Input: dimensioned drawing with shaded views. Units: mm. Origin: part minimum x, y, z. Round coordinates to 2 decimals unless told otherwise and drop trailing zeros. Order: outer loops, then holes, each group sorted by start corner. A loop starts at its lowest first (then second) coordinate and runs counter-clockwise, first axis right, second up. Notation, with made-up numbers: M 25,88.25 L 82,88.25 A29 ccw 82,125.25 Z; hole C 57,33.25 d5. An arc over 180 degrees is marked long. Use one line per item in the form item = value. Start each with the question number.
Q1. Material intervals for probe 1 along Z at (x, y) = (123, 2.15); probe 2 along Z at (x, y) = (79, 1.2) (1 decimal); probe 3 along X at (y, z) = (2.5, 35.5) (1 decimal), sorted ascending.
Q2. Section A-A (z = 95.25). Give the number of separate pieces and of enclosed holes in the cut face, plus the area to 3 significant figures.
Q3. Contact query for flat-ended pins moving along their axis: pin 1 (1 mm diameter, centred on x = 131.5, y = 2, fed in from -Z); pin 2 (1.6 mm diameter, centred on y = 1.5, z = 70, fed in from -X) (3 decimals); pin 3 (1 mm diameter, centred on x = 2, y = 2, fed in from +Z). Output: stop coordinate, or through.
Q4. Section B-B (x = 59). Return the cut outline in (y, z) (1 decimal).
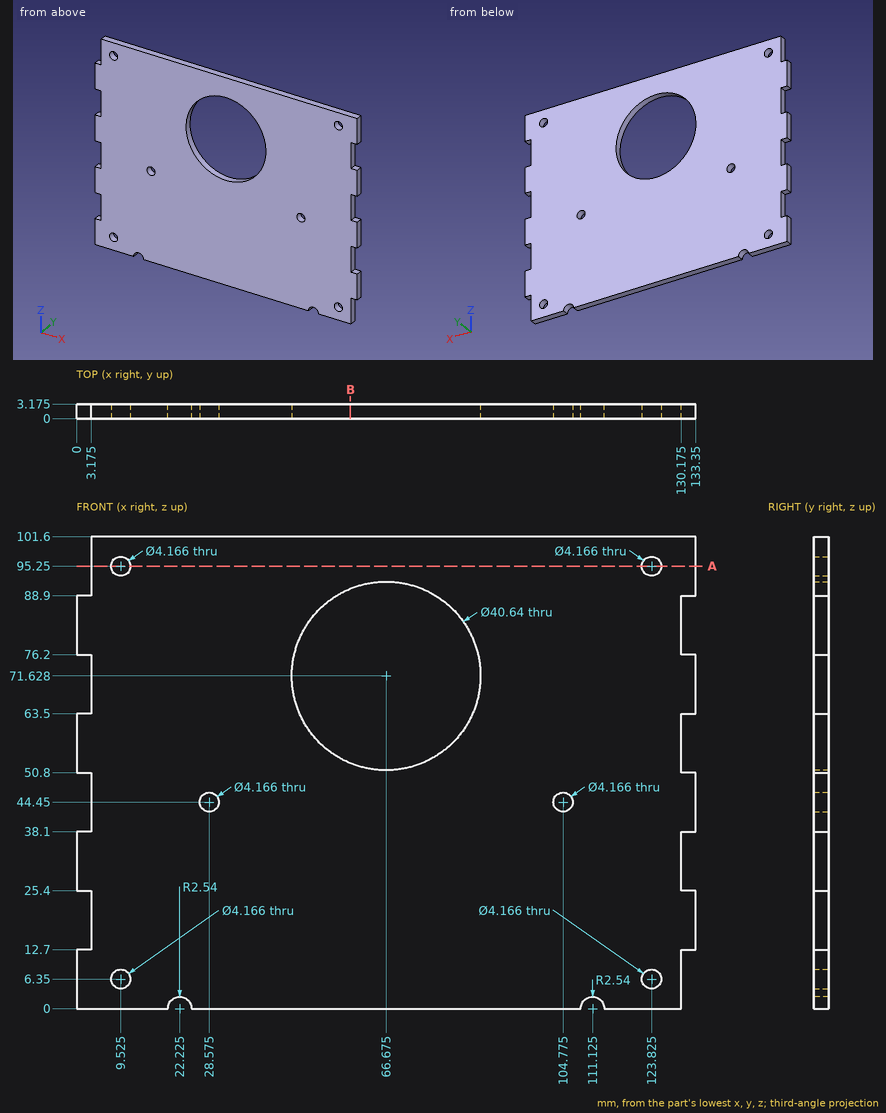
Results list:
q1.probe_1 = 0 to 4.44, 8.26 to 93.34, 97.16 to 101.6
q1.probe_2 = 0 to 55.5, 87.8 to 101.6
q1.probe_3 = 0 to 130.2
q2.separate_pieces = 3
q2.enclosed_holes = 0
q2.area = 387 mm2
q3.pin_1 = 12.7
q3.pin_2 = 3.175
q3.pin_3 = 88.9
q4.outline = M 0,0 L 3.2,0 L 3.2,52.8 L 0,52.8 Z; M 0,90.4 L 3.2,90.4 L 3.2,101.6 L 0,101.6 Z
